Check sheet for the drawn part. Datum: minimum x, y, z corner. Units: mm. A direction names the side the tool comes from. Round coordinates to 2 decimals unless told otherwise and drop trailing zeros. Write each loop counter-clockwise with the first axis right and the second up, starting at its lowest first coordinate (ties: lowest second). Pieces come first, ordered by that corner, then holes. Notation, with made-up numbers: (-4, 28.25) -> (5, 28.25) arc R17 cw to (5, 46.25) -> close; hole circle Ø3 at (18, 40.5). An arc over 180 degrees is marked (long way). One line per item, written item: value.
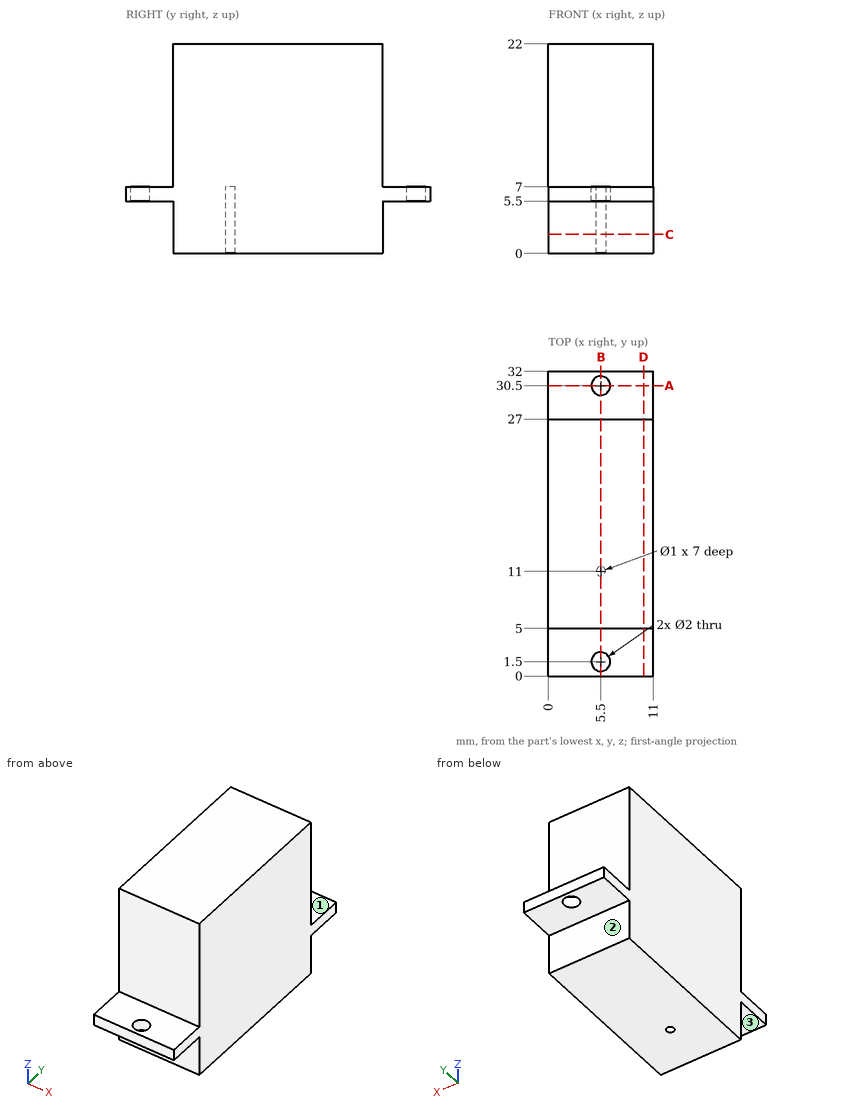
Item 1: Sectioned sample at C-C on z = 2. Enter the section's corners in (x, y).
Answer:
outline: (0, 5) -> (11, 5) -> (11, 27) -> (0, 27) -> close; hole circle Ø1 at (5.5, 11)
Item 2: Sectioned sample at A-A on y = 30.5. Enter the section's corners in (x, z).
Answer:
outline: (0, 5.5) -> (4.5, 5.5) -> (4.5, 7) -> (0, 7) -> close; (6.5, 5.5) -> (11, 5.5) -> (11, 7) -> (6.5, 7) -> close
Item 3: Sectioned sample at B-B on x = 5.5. Enter the section's corners in (y, z), and give its area (3 significant figures).
Answer:
outline: (0, 5.5) -> (0.5, 5.5) -> (0.5, 7) -> (0, 7) -> close; (2.5, 5.5) -> (5, 5.5) -> (5, 0) -> (10.5, 0) -> (10.5, 7) -> (11.5, 7) -> (11.5, 0) -> (27, 0) -> (27, 5.5) -> (29.5, 5.5) -> (29.5, 7) -> (27, 7) -> (27, 22) -> (5, 22) -> (5, 7) -> (2.5, 7) -> close; (31.5, 5.5) -> (32, 5.5) -> (32, 7) -> (31.5, 7) -> close
area: 486 mm^2
Item 4: Tool access check on the marked faces 1, 2 and 3. Record the directions out of +Z, -Z, +X, -X, +Y, -Y that give a thin tool (end or side, any length) a straight path to the whole face; none if there is none.
Answer:
face 1: +Z, +X, -X, +Y
face 2: -Z, +X, -X, +Y
face 3: -Z, +X, -X, -Y
Item 5: Sectioned sample at D-D on x = 10. Enter the section's corners in (y, z), and give its area (3 significant figures).
Answer:
outline: (0, 5.5) -> (5, 5.5) -> (5, 0) -> (27, 0) -> (27, 5.5) -> (32, 5.5) -> (32, 7) -> (27, 7) -> (27, 22) -> (5, 22) -> (5, 7) -> (0, 7) -> close
area: 499 mm^2
Item 6: Thickness scan on line 1 (Y direction, x = 5.5, z = 6.05); line 2 (Y direction, x = 6, z = 10); line 3 (Z direction, x = 5.5, y = 4). Record the ranges inside material, lowest first.
Answer:
line 1: y = 0 to 0.5, 2.5 to 10.5, 11.5 to 29.5, 31.5 to 32
line 2: y = 5 to 27
line 3: z = 5.5 to 7
Item 7: Depth check by flat-ended pin: P1, Ø1.8, axis at x = 5.5, y = 1.5, coming from the -Z side; P2, Ø5.5, axis at x = 3, z = 15, coming from the +Y side; P3, Ø4, axis at x = 6, y = 2.5, coming from the -Z side; P4, Ø1.6, axis at x = 7, z = 2, coming from the -Y side. Enter the tip coordinate at first touch or a pass-through.
Answer:
P1: passes through
P2: stops at y = 27
P3: stops at z = 5.5
P4: stops at y = 5
